from build123d import *

# Parameters (mm, degrees)
SKETCH1_R           = 10
BOSS_EXTRUDE1_DEPTH = 1.5
SKETCH2_R           = 1.4
CUT_EXTRUDE1_DEPTH  = 2.5
SKETCH3_R           = 3.5
BOSS_EXTRUDE2_DEPTH = 3.5
FILLET1_R           = 0.5


with BuildPart() as part:
    # Sketch1 → Boss-Extrude1 (new body)
    with BuildSketch(Plane(origin=(0, 0, 0), x_dir=(1, 0, 0), z_dir=(0, 1, 0))):
        Circle(SKETCH1_R)
    extrude(amount=-BOSS_EXTRUDE1_DEPTH)

    # Sketch2 → Cut-Extrude1 (cut, through all)
    with BuildSketch(Plane(origin=(0, 0, 0), x_dir=(1, 0, 0), z_dir=(0, 1, 0))):
        with Locations((0, 7)):
            Circle(SKETCH2_R)
        with Locations((0, -7)):
            Circle(SKETCH2_R)
    extrude(amount=-CUT_EXTRUDE1_DEPTH, mode=Mode.SUBTRACT)

    # Sketch3 → Boss-Extrude2 (add)
    with BuildSketch(Plane.XZ.offset(1.5)):
        Circle(SKETCH3_R)
        with BuildLine():
            Line((1.985734783, 1.647196822), (2.166931392, -1.400288664))
            ThreePointArc((2.166931392, -1.400288664), (-2.575451618, -0.15313054), (1.985734783, 1.647196822))
        make_face(mode=Mode.SUBTRACT)
    extrude(amount=BOSS_EXTRUDE2_DEPTH)

    # Fillet1
    fillet1_edges = [part.edges().sort_by_distance(p)[0] for p in [
        (-2.575451618, -5, -0.15313054),
        (2.076333088, -5, 0.123454079),
    ]]
    fillet(fillet1_edges, radius=FILLET1_R)


solid = part.part
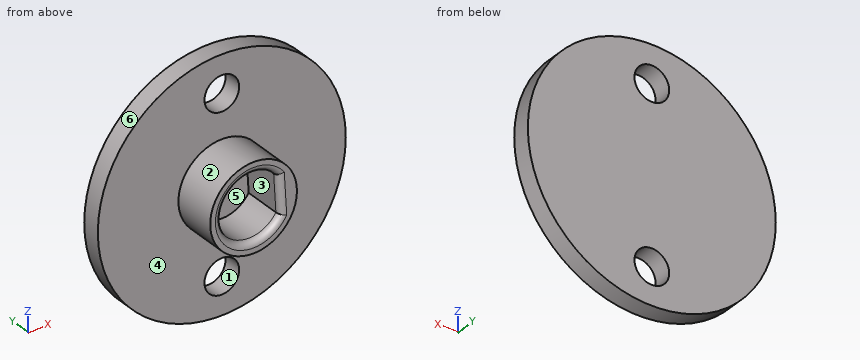
Read the model definition and answer for the solid it produces. Units are mm, in the model's axes. Face numbers are marked on the shaded views. A direction names the side the tool comes from. Coordinates: 2 decimals unless noted, no trailing zeros. Order: outer loops, then holes, each group sorted by start corner. A loop starts at its lowest first (then second) coordinate and runs counter-clockwise, first axis right, second up. Notation, with made-up numbers: M 57,-14 L 97,-14 A24 ccw 97,17 Z; hole C -13,76 d4. An arc over 180 degrees is marked long. Put each result on its own line as item: value. Start each with the question number.
Item 1: Section C-C, the plane y = -4.25 is taken. Determine the outline of the cut face in (x, z).
Item 2: Section D-D, the plane x = -8 is taken. Determine the outline of the cut face in (y, z), plus the area to 3 significant figures.
Item 3: Given pin 1 Ø1.5 at (y, z) = (-2.5, -7.5) entering from -X; pin 2 Ø2.5 at (x, z) = (0.5, 1.5) entering from -Y, each flat-ended and moving along its own axis, determine where each tip first touches the part or whether it passes through.
Item 4: For the marked faces 5 and 6, determine the directions among +Z, -Z, +X, -X, +Y, -Y from which every point of the face is accessible in a straight line to the end or side of a thin tool.
Item 5: Section B-B, the plane x = 0 is taken. Count the separate pieces of the cut face and the enclosed holes in it, plus the area to 3 significant figures.
Item 6: Section A-A, the plane z = 7.5 is taken. Determine the outline of the cut face in (x, y), plus the area to 3 significant figures.
Item 7: Consider probe 1 along Z at (x, y) = (0, -1.05); probe 2 along Z at (x, y) = (0, -2.75); probe 3 along Z at (x, y) = (-1.25, -0.7). Determine where each line is inside the solid, lowest interval first. Write a range as [from, to].
Item 8: The mould has two halves that part along X. Classify the marked faces 1, 2, 3 and 4: +X half, -X half, draft (parallel to the pull), parting line (faces both ways), or undercut.
Computed:
1. outline: C 0,0 d7; hole M 1.99,1.65 A2.58 ccw long 2.17,-1.4 Z
2. outline: M -1.5,-6 L 0,-6 L 0,6 L -1.5,6 Z
2. area: 18.0 mm2
3. pin 1: passes through
3. pin 2: stops at y = -4.93
4. face 5: -Y
4. face 6: +Y, -Y
5. separate pieces: 3
5. enclosed holes: 0
5. area: 27.9 mm2
6. outline: M -6.61,-1.5 L -1.31,-1.5 L -1.31,0 L -6.61,0 Z; M 1.31,-1.5 L 6.61,-1.5 L 6.61,0 L 1.31,0 Z
6. area: 15.9 mm2
7. probe 1: z = [-10, -8.4], [-5.6, 5.6], [8.4, 10]
7. probe 2: z = [-3.5, -2.58], [2.58, 3.5]
7. probe 3: z = [-9.92, -7.63], [-6.37, 6.37], [7.63, 9.92]
8. face 1: undercut
8. face 2: parting line
8. face 3: undercut
8. face 4: draft
